Build history of the part. All positions in model axes, mm. A direction names the side the tool comes from. Give positions to 0.01 mm unless a question says otherwise; leave off trailing zeros. Loops run counter-clockwise (first coordinate to the right, second up) from the corner with the lowest first, then second, coordinate; pieces in that order, holes last.
1) 3-axis set-ups, long thin cutter, end or side, ignore diameter. For faces 1 (the flat face through (-1, 0, 0)), 2 (the flat face through (39, 5, 0)), 3 (the flat face through (-48, 15, 28)): which of +Z, -Z, +X, -X, +Y, -Y reach the whole face in a straight line?
2) Band-saw the part on C-C on z = 0. List the corners of the cut face in (x, y), then the cut area to 4 significant figures.
3) Band-saw the part on B-B on x = -29.5. List the corners of the cut face in (y, z), then the cut area to 3 significant figures.
4) Band-saw the part on D-D on x = 9. List the corners of the cut face in (y, z), then the cut area to 3 significant figures.
5) Band-saw the part on A-A on y = 12.25. List the corners of the cut face in (x, z), then the cut area to 3 significant figures.
6) Two-plate mould, pull along Z, no slides. Class faces 4 (the flat face through (-48, 25, 29)), 5 (the flat face through (-81.5, 15, 0)), 6 (the flat face through (-48, 15, -28)), 7 (the flat face through (-40, 10, -33)): +Z half, -Z half, draft (parallel to the pull), parting line (faces both ways), or undercut.
7) Flat gauge pins, fed straight in: P1, Ø2, axis at x = 43.5, z = -18, coming from the +Y side; P2, Ø10, axis at y = 14.5, z = -5.5, coming from the +X side. Where does each tip first touch, or does it go through?
8) Wall check: line 1 (Z direction, x = -34.5, y = 10.75); line 2 (X direction, y = 20, z = -22); line 3 (X direction, y = 22.5, z = 30.5). Give the ranges that are in metal, low to high.
```python
from build123d import *

# Parameters (mm, degrees)
SKETCH1_W           = 173
SKETCH1_H           = 66
BOSS_EXTRUDE1_DEPTH = 5
SKETCH3_W           = 78.9
SKETCH3_H           = 66
BOSS_EXTRUDE2_DEPTH = 20
SHELL1_T            = -5


with BuildPart() as part:
    # Sketch1 → Boss-Extrude1 (new body)
    with BuildSketch(Plane(origin=(0, 0, 0), x_dir=(1, 0, 0), z_dir=(0, 1, 0))):
        Rectangle(SKETCH1_W, SKETCH1_H)
    extrude(amount=BOSS_EXTRUDE1_DEPTH)

    # Sketch3 → Boss-Extrude2 (add)
    with BuildSketch(Plane(origin=(0, 5, 0), x_dir=(1, 0, 0), z_dir=(0, 1, 0))):
        with Locations((-47.05, 0)):
            Rectangle(SKETCH3_W, SKETCH3_H)
    extrude(amount=BOSS_EXTRUDE2_DEPTH)

    # Shell1
    shell1_openings = [part.faces().sort_by_distance(p)[0] for p in [
        (-47.05, 25, 0),
    ]]
    offset(amount=SHELL1_T, openings=shell1_openings, kind=Kind.INTERSECTION)


solid = part.part
```
Findings below:
1. face 1: +Z, -Z, +X, -X, -Y
1. face 2: +Z, -Z, +X, +Y
1. face 3: +Y
2. outline: (-86.5, 0) - (86.5, 0) - (86.5, 5) - (-7.6, 5) - (-7.6, 25) - (-12.6, 25) - (-12.6, 5) - (-81.5, 5) - (-81.5, 25) - (-86.5, 25) - close
2. area: 1,065 mm2
3. outline: (0, -33) - (25, -33) - (25, -28) - (5, -28) - (5, 28) - (25, 28) - (25, 33) - (0, 33) - close
3. area: 530 mm2
4. outline: (0, -33) - (5, -33) - (5, 33) - (0, 33) - close
4. area: 330 mm2
5. outline: (-86.5, -33) - (-7.6, -33) - (-7.6, 33) - (-86.5, 33) - close; hole (-81.5, -28) - (-12.6, -28) - (-12.6, 28) - (-81.5, 28) - close
5. area: 1,350 mm2
6. face 4: draft
6. face 5: undercut
6. face 6: undercut
6. face 7: -Z half
7. P1: stops at y = 5
7. P2: stops at x = -7.6
8. line 1: z = -33 to -28, 28 to 33
8. line 2: x = -86.5 to -81.5, -12.6 to -7.6
8. line 3: x = -86.5 to -7.6
